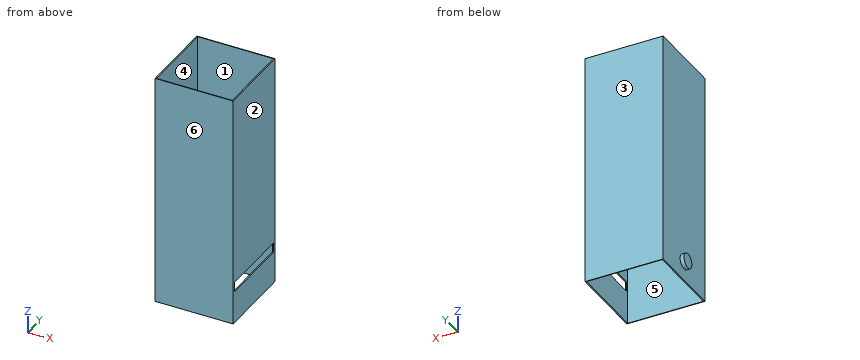
from build123d import *

# Parameters (mm, degrees)
F0_W     = 101.6
F0_H     = 304.8
F1_DEPTH = 50.8
F2_W     = 98.425
F2_H     = 100.000558
F3_DEPTH = 304.8
F4_W     = 95.25
F4_H     = 12.7
F5_DEPTH = 25.4
F6_R     = 9.525
F7_DEPTH = 5.08
F8_R     = 0.612831
F9_DEPTH = 0.254


with BuildPart() as f1:
    # F0 (on Front) → F1 (new body, symmetric)
    with BuildSketch(Plane.XZ):
        Rectangle(F0_W, F0_H)
    extrude(amount=F1_DEPTH, both=True)

    # F2 (on face) → F3 (cut)
    with BuildSketch(Plane.XY.offset(152.4)):
        Rectangle(F2_W, F2_H)
    extrude(amount=-F3_DEPTH, mode=Mode.SUBTRACT)

    # F4 (on face) → F5 (cut)
    with BuildSketch(Plane.YZ.offset(50.8)):
        with Locations((0, -103.808521)):
            Rectangle(F4_W, F4_H)
    extrude(amount=-F5_DEPTH, mode=Mode.SUBTRACT)

    # F6 (on face) → F7 (join)
    with BuildSketch(Plane(origin=(-50.8, 0, 0), x_dir=(0, -1, 0), z_dir=(-1, 0, 0))):
        with Locations((0, -127.594535)):
            Circle(F6_R)
    extrude(amount=F7_DEPTH)

    # F8 (on face) → F9 (cut)
    with BuildSketch(Plane.YZ.offset(-49.2125)):
        with Locations((0, -103.871576)):
            Circle(F8_R)
    extrude(amount=-F9_DEPTH, mode=Mode.SUBTRACT)


solid = f1.part
Read the model definition and answer for the solid it produces. Units are mm, in the model's axes. Face numbers are marked on the shaded views. A direction names the side the tool comes from. Give positions to 0.01 mm unless a question says otherwise; leave off trailing zeros. Write each loop counter-clockwise with the first axis right and the second up, starting at its lowest first coordinate (ties: lowest second). Pieces come first, ordered by that corner, then holes. Notation, with made-up numbers: (35.5, 78) -> (66.5, 78) arc R23 cw to (66.5, 116) -> close; hole circle Ø7 at (-4.5, 52). An arc over 180 degrees is marked (long way). Answer as a JSON object with one key per item and string values. Group by question number.
1) Find section A-A (y = -40.5). Write down the section's boundary in (x, z), and give its area (3 significant figures).
2) A tool of negligible diameter and unlimited length cuts with its end or side. For the marked faces 5 and 6, from which of +Z, -Z, +X, -X, +Y, -Y can it reach the whole face along a straight path? Write none if from no direction.
3) Consider L1, parallel to Y at x = -13.5, z = 54.5; L2, parallel to X at y = -16.5, z = -133.5; L3, parallel to Z at x = -49.25, y = 0. Determine where each line is inside the solid, lowest interval first. Write a range as from..to.
4) Find section C-C (z = 11). Write down the section's boundary in (x, y), and give its area (3 significant figures).
5) The mould has two halves that part along X. Classify the marked faces 1, 2, 3 and 4: +X half, -X half, draft (parallel to the pull), parting line (faces both ways), or undercut.
6) This flat-tipped pin is pushed along its axis until it touches: P1, Ø12, axis at y = 3.5, z = 17.5, coming from the -X side. Where does it stop, or does it pass through?
7) Find section B-B (x = 13). Write down the section's boundary in (y, z).
Values follow:
{
 "1": {"outline": "(-50.8, -152.4) -> (-49.21, -152.4) -> (-49.21, 152.4) -> (-50.8, 152.4) -> close; (49.21, -152.4) -> (50.8, -152.4) -> (50.8, -110.16) -> (49.21, -110.16) -> close; (49.21, -97.46) -> (50.8, -97.46) -> (50.8, 152.4) -> (49.21, 152.4) -> close", "area": "948 mm2"},
 "2": {"face 5": "+Z, -Z", "face 6": "+Z, -Z, +X, -X, -Y"},
 "3": {"L1": "y = -50.8..-50, 50..50.8", "L2": "x = -50.8..-49.21, 49.21..50.8", "L3": "z = -152.4..-104.48, -103.26..152.4"},
 "4": {"outline": "(-50.8, -50.8) -> (50.8, -50.8) -> (50.8, 50.8) -> (-50.8, 50.8) -> close; hole (-49.21, -50) -> (49.21, -50) -> (49.21, 50) -> (-49.21, 50) -> close", "area": "480 mm2"},
 "5": {"face 1": "undercut", "face 2": "+X half", "face 3": "draft", "face 4": "undercut"},
 "6": {"P1": "stops at x = -50.8"},
 "7": {"outline": "(-50.8, -152.4) -> (-50, -152.4) -> (-50, 152.4) -> (-50.8, 152.4) -> close; (50, -152.4) -> (50.8, -152.4) -> (50.8, 152.4) -> (50, 152.4) -> close"}
}
